Work out the finished part from the listing and answer in its coordinate system (mm). A direction names the side the tool comes from. Round coordinates to 2 decimals unless told otherwise and drop trailing zeros. Write each loop counter-clockwise with the first axis right and the second up, starting at its lowest first coordinate (ties: lowest second). Pieces come first, ordered by that corner, then holes. Notation, with made-up numbers: (11, 18) -> (19, 18) arc R28 ccw to (19, 57) -> close; hole circle Ø8 at (-12.75, -33). An arc over 180 degrees is marked (long way). One line per question, with ' | ' between items. Start each with the question number.
```python
from build123d import *

# Parameters (mm, degrees)
F1_DEPTH = 10
F2_R     = 2
F3_R     = 1.4
F4_DEPTH = 11
F3_R_2   = 2.85
F5_DEPTH = 2


with BuildPart() as f1:
    # F0 (on Top) → F1 (new body)
    with BuildSketch(Plane.XY):
        with BuildLine():
            ThreePointArc((77.2961207269, 6.3033039919), (74.9125256302, 5.3313144616), (72.3597780987, 5))
            Line((72.3597780987, 5), (0, 5))
            Line((0, 5), (0, -5))
            Line((0, -5), (71.6958680115, -5))
            ThreePointArc((71.6958680115, -5), (74.8331804116, -4.495118267), (77.6536984673, -3.0314541808))
            Line((77.6536984673, -3.0314541808), (87.9106565848, 4.5772821801))
            ThreePointArc((87.9106565848, 4.5772821801), (89.3979800506, 6.3451854495), (89.9317413568, 8.5930092705))
            Line((89.9317413568, 8.5930092705), (89.9317413568, 10.0404781398))
            ThreePointArc((89.9317413568, 10.0404781398), (88.9380869607, 11.7688497797), (86.9444728312, 11.7798173414))
            Line((86.9444728312, 11.7798173414), (77.2961207269, 6.3033039919))
        make_face()
    extrude(amount=F1_DEPTH)

    # F2
    f2_edges = [f1.edges().sort_by_distance(p)[0] for p in [
        (35.847934, -5, 10),
        (35.847934, -5, 0),
    ]]
    fillet(f2_edges, radius=F2_R)

    # F3 (on face) → F4 (cut)
    with BuildSketch(Plane.XZ.offset(5)):
        with Locations((61.6958680115, 5)):
            Circle(F3_R)
    extrude(amount=-F4_DEPTH, mode=Mode.SUBTRACT)

    # F3 (on face) → F5 (cut)
    with BuildSketch(Plane.XZ.offset(5)):
        with Locations((61.6958680115, 5)):
            Circle(F3_R_2)
        with Locations((61.6958680115, 5)):
            Circle(F3_R, mode=Mode.SUBTRACT)
    extrude(amount=-F5_DEPTH, mode=Mode.SUBTRACT)

    # F6: F1 across plane


with BuildPart() as f1_1:
    add(f1.part)
    add(f1.part.mirror(Plane.YZ))


solid = f1_1.part
```
(1) A cutting plane is placed at A-A, the plane x = -3. Determine the outline of the cut face in (y, z), then the cut area to 3 significant figures.
(2) The mould has two halves that part along X. Classify faces 1 (the flat face through (1, -5, 5)), 2 (the flat face through (82.71, 0.72, 4.96)), 3 (the cylindrical face through (-74.95, 5.34, 4.96)): +X half, -X half, draft (parallel to the pull), parting line (faces both ways), or undercut.
(3) Given pin 1 Ø2 at (y, z) = (2.5, 2.5) entering from -X; pin 2 Ø4.5 at (x, z) = (61.5, 4.5) entering from -Y; pin 3 Ø3 at (x, z) = (36.5, 9) entering from +Y; pin 4 Ø2 at (x, z) = (61.7, 5) entering from +Y, each flat-ended and moving along its own axis, determine where each tip first touches the part or whether it passes through.
(4) Consider L1, parallel to X at y = -4, z = 6.25; L2, parallel to Y at x = -45, z = 6.5; L3, parallel to X at y = 11.5, z = 3.75. Determine where each line is inside the solid, lowest interval first.
(5) A cutting plane is placed at B-B, the plane y = 1.25. Count the separate pieces of the cut face and the enclosed holes in it, then the cut area to 3 significant figures.
(6) For faces 4 (the cylindrical face through (64.4, -4, 5.9)), 5 (the cylindrical face through (89.383, 6.316, 4.958)), 6 (the flat face through (1, 1, 0)), 7 (the flat face through (82.19, 9.08, 4.96)), 8 (the cylindrical face through (82.334, 8.507, 9.399)), determine the directions among +Z, -Z, +X, -X, +Y, -Y from which every point of the face is accessible in a straight line to the end or side of a thin tool.
Returned:
1) outline: (-5, 2) arc R2 ccw to (-3, 0) -> (3, 0) arc R2 ccw to (5, 2) -> (5, 8) arc R2 ccw to (3, 10) -> (-3, 10) arc R2 ccw to (-5, 8) -> close | area: 96.6 mm2
2) face 1: draft | face 2: +X half | face 3: undercut
3) pin 1: x = -86.46 | pin 2: y = -3 | pin 3: y = 5 | pin 4: through
4) L1: -76.05 to -64.26, -59.13 to 59.13, 64.26 to 76.05 | L2: -5 to 5 | L3: -89.3 to -86.45, 86.45 to 89.3
5) separate pieces: 1 | enclosed holes: 2 | area: 1,650 mm2
6) face 4: -Y | face 5: +Z, -Z, +X, -Y | face 6: -Z, +X, -X, +Y, -Y | face 7: +Z, -Z, +Y | face 8: +Z, +Y
